Could you check a few things on this model? Use its own coordinates, in mm. Coordinates: 2 decimals unless noted, no trailing zeros. Order: outer loops, then holes, each group sorted by start corner. A loop starts at its lowest first (then second) coordinate and runs counter-clockwise, first axis right, second up. Notation, with made-up numbers: (-39, 29.25) - (11, 29.25) arc R13 cw to (11, 38.25) - close; hole circle Ø5 at (-15.75, -13.5). An arc over 180 degrees is marked (long way). Answer as CSV lines item,"result". Start each with the question number.
1. I want a section at A-A, the plane z = -564. List the corners of the cut face in (x, y) for me, and give its area (3 significant figures).
2. I need wall thicknesses on probe 1 along X at (y, z) = (106.5, 26); probe 2 along Z at (x, y) = (787.4, -301); probe 3 along X at (y, z) = (232.5, 62.5). Which ranges of each line are inside material? Lowest first, please.
3. I want a section at B-B, the plane x = -576.5. List the corners of the cut face in (y, z) for me, and give its area (3 significant figures).
4. For pin 1 (15 mm diameter, centred on x = 792.5, z = -272, fed in from +Y); pin 2 (3 mm diameter, centred on x = 401.5, y = -133, fed in from -Z); pin 3 (8 mm diameter, centred on x = 20, y = 18, fed in from +Z); pin 4 (8.5 mm diameter, centred on x = -787.4, z = 25.4, fed in from -Y), each with a flat end and sliding along its axis, tell me the tip position at first contact or that it passes through.
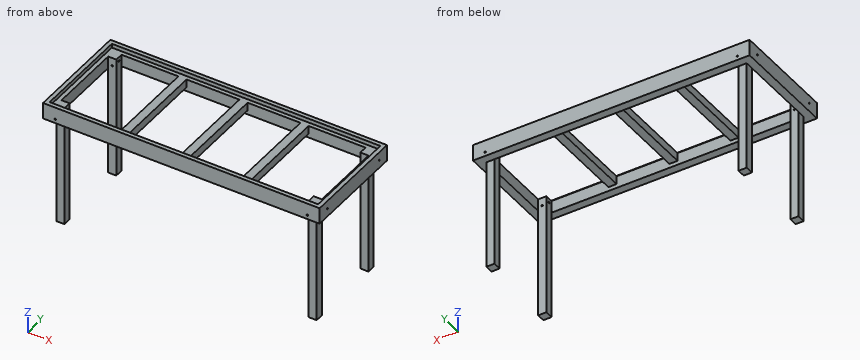
from build123d import *

# Parameters (mm, degrees)
F0_W          = 1727.2
F0_H          = 660.4
F0_W_2        = 1676.4
F0_H_2        = 609.6
F1_DEPTH      = 101.6
F2_W          = 1676.4
F2_H          = 609.6
F2_W_2        = 1625.6
F2_H_2        = 558.8
F3_DEPTH      = 76.2
F4_W          = 50.8
F4_H          = 50.8
F5_DEPTH      = 76.2
F5_DEPTH_BACK = 685.8
F6_R          = 4.7625
F7_DEPTH      = 1727.201
F8_R          = 4.7625
F9_DEPTH      = 660.401
F10_W         = 50.8
F10_H         = 558.8
F11_DEPTH     = 50.8


with BuildPart() as f1:
    # F0 (on Top) → F1 (new body)
    with BuildSketch(Plane.XY):
        Rectangle(F0_W, F0_H)
        Rectangle(F0_W_2, F0_H_2, mode=Mode.SUBTRACT)
    extrude(amount=F1_DEPTH)

    # F2 (on Top) → F3 (join)
    with BuildSketch(Plane.XY):
        Rectangle(F2_W, F2_H)
        Rectangle(F2_W_2, F2_H_2, mode=Mode.SUBTRACT)
    extrude(amount=F3_DEPTH)

    # F4 (on Top) → F5 (join, two sides)
    with BuildSketch(Plane.XY) as f5_sk:
        with Locations((-787.4, -254)):
            Rectangle(F4_W, F4_H)
        with Locations((-787.4, 254)):
            Rectangle(F4_W, F4_H)
        with Locations((787.4, -254)):
            Rectangle(F4_W, F4_H)
        with Locations((787.4, 254)):
            Rectangle(F4_W, F4_H)
    extrude(amount=F5_DEPTH)
    extrude(f5_sk.sketch, amount=-F5_DEPTH_BACK)

    # F6 (on face) → F7 (cut, through all)
    with BuildSketch(Plane.YZ.offset(863.6)):
        with Locations((-254, 50.8)):
            Circle(F6_R)
        with Locations((254, 50.8)):
            Circle(F6_R)
    extrude(amount=-F7_DEPTH, mode=Mode.SUBTRACT)

    # F8 (on face) → F9 (cut, through all)
    with BuildSketch(Plane.XZ.offset(330.2)):
        with Locations((-787.4, 25.4)):
            Circle(F8_R)
        with Locations((787.4, 25.4)):
            Circle(F8_R)
    extrude(amount=-F9_DEPTH, mode=Mode.SUBTRACT)

    # F10 (on face) → F11 (join)
    with BuildSketch(Plane.XY.offset(76.2)):
        with Locations((-381, 0)):
            Rectangle(F10_W, F10_H)
        with Locations((381, 0)):
            Rectangle(F10_W, F10_H)
        Rectangle(F10_W, F10_H)
    extrude(amount=-F11_DEPTH)


solid = f1.part
Solved:
1,outline,"(-812.8, -279.4) - (-762, -279.4) - (-762, -228.6) - (-812.8, -228.6) - close; (-812.8, 228.6) - (-762, 228.6) - (-762, 279.4) - (-812.8, 279.4) - close; (762, -279.4) - (812.8, -279.4) - (812.8, -228.6) - (762, -228.6) - close; (762, 228.6) - (812.8, 228.6) - (812.8, 279.4) - (762, 279.4) - close"
1,area,"10,300 mm2"
2,probe 1,"x = -863.6 to -812.8, -406.4 to -355.6, -25.4 to 25.4, 355.6 to 406.4, 812.8 to 863.6"
2,probe 2,"z = 0 to 20.64, 30.16 to 76.2"
2,probe 3,"x = -863.6 to -762, -406.4 to -355.6, -25.4 to 25.4, 355.6 to 406.4, 762 to 863.6"
3,outline,"(-330.2, 0) - (-279.4, 0) - (-279.4, 76.2) - (-304.8, 76.2) - (-304.8, 101.6) - (-330.2, 101.6) - close; (279.4, 0) - (330.2, 0) - (330.2, 101.6) - (304.8, 101.6) - (304.8, 76.2) - (279.4, 76.2) - close"
3,area,"9,030 mm2"
4,pin 1,"stops at y = 279.4"
4,pin 2,"stops at z = 25.4"
4,pin 3,"stops at z = 76.2"
4,pin 4,"passes through"
